Verification items for the finished model (mm, model axes). A direction names the side the tool comes from. Round coordinates to 2 decimals unless told otherwise and drop trailing zeros. Order: outer loops, then holes, each group sorted by start corner. A loop starts at its lowest first (then second) coordinate and runs counter-clockwise, first axis right, second up. Notation, with made-up numbers: M 36.25,48.25 L 66.25,48.25 A32 ccw 66.25,82.25 Z; hole C 62.25,41.25 d5. An arc over 180 degrees is marked long. Use one line per item in the form item = value. Start each with the question number.
Item 1: Tool access check on faces 1 (the flat face through (-5, -2.54, 1)), 2 (the flat face through (-22.972, -2.576, -0.787)), 3 (the flat face through (-3.175, -1, 0)). Record the directions out of +Z, -Z, +X, -X, +Y, -Y that give a thin tool (end or side, any length) a straight path to the whole face; none if there is none.
Item 2: Cross-section at A-A on z = -1.5. Enter the section's corners in (x, y) (3 decimals), then the cut area to 3 significant figures.
Item 3: Cross-section at B-B on y = -1.65. Enter the section's corners in (x, z) (1 decimal).
Item 4: Cross-section at C-C on x = -13.5. Enter the section's corners in (y, z), then the cut area to 3 significant figures.
Item 5: Cross-section at D-D on z = -24. Enter the section's corners in (x, y), then the cut area to 3 significant figures.
Item 6: Thickness scan on probe 1 along Y at (x, z) = (-6.5, 29); probe 2 along Z at (x, y) = (-2.5, -1.45) (3 decimals); probe 3 along Z at (x, y) = (-1, -2.85). Record the ranges inside material, lowest first. Write a range as [from, to].
Item 7: Go/stop test with flat-tipped pins: pin 1 Ø1.5 at (y, z) = (-2, 18) entering from -X; pin 2 Ø3 at (x, y) = (-1, -1.5) entering from -Z; pin 3 Ø1 at (x, y) = (-11, -1.5) entering from +Z. Record where each tip stops, or that it passes through.
Item 8: Release check for a two-part mould opening along Z. For faces 4 (the flat face through (-0.432, -2.576, 48.22)), 5 (the flat face through (-5, 0, 1)), 6 (the flat face through (-0.432, -2.576, -48.372)), 7 (the conical face through (19.4, -4.1, 44.8)) record: +Z half, -Z half, draft (parallel to the pull), parting line (faces both ways), or undercut.
from build123d import *

# Parameters (mm, degrees)
F0_W        = 50.8
F0_H        = 101.6
F0_R        = 1.143
F0_R_2      = 1.2394927364
F1_DEPTH    = 5.08
F2_T1_DEPTH = 127.7282991577
F2_T3_DEPTH = 76.9282991577
F3_T        = -2.54
F4_W        = 6.35
F4_H        = 19.05
F5_DEPTH    = 25.4


# Not quite as in the source:
# - a fillet or chamfer that OpenCascade refuses, or shapes differently, is made with other operations: its cross-section is extruded or revolved along the edge and cut away or added


with BuildPart() as f1:
    # F0 (on Front) → F1 (new body)
    with BuildSketch(Plane.XZ):
        with Locations((-0.076776122, -0.0760140894)):
            Rectangle(F0_W, F0_H)
        with Locations((-22.936776122, -48.2090140894)):
            Circle(F0_R, mode=Mode.SUBTRACT)
        with Locations((23.418223878, -49.0980140894)):
            Circle(F0_R, mode=Mode.SUBTRACT)
        with Locations((-23.6282116387, 48.9378400757)):
            Circle(F0_R_2, mode=Mode.SUBTRACT)
        with Locations((23.5306444928, 48.7492585503)):
            Circle(F0_R, mode=Mode.SUBTRACT)
    extrude(amount=F1_DEPTH)

    # F2: chamfer of 5.08 on 8 edges, made by hand

    # F2_s2 → F2_t1 (cut)
    with BuildSketch(Plane.XY.offset(-63.9401636683)):
        Polygon((25.323223878, -5.08), (20.243223878, 0), (25.323223878, 0), align=None)
        Polygon((-25.476776122, -5.08), (-20.396776122, 0), (-25.476776122, 0), align=None)
    extrude(amount=F2_T1_DEPTH, mode=Mode.SUBTRACT)

    # F2_s4 → F2_t3 (cut)
    with BuildSketch(Plane.YZ.offset(-38.5409257009)):
        Polygon((-5.08, 50.7239859106), (0, 45.6439859106), (0, 50.7239859106), align=None)
        Polygon((-5.08, -50.8760140894), (0, -45.7960140894), (0, -50.8760140894), align=None)
    extrude(amount=F2_T3_DEPTH, mode=Mode.SUBTRACT)

    # F2_s5 → F2_t6 (revolve, cut)
    with BuildSketch(Plane.XY.offset(48.9378400757)):
        Polygon((-22.3887189023, -5.08), (-17.3087189023, 0), (-22.3887189023, 0), align=None)
    revolve(axis=Axis((-23.6282116387, 0, 48.9378400757), (0, -1, 0)), mode=Mode.SUBTRACT)

    # F2_s7 → F2_t8 (revolve, cut)
    with BuildSketch(Plane.XY.offset(48.7492585503)):
        Polygon((24.6736444928, -5.08), (29.7536444928, 0), (24.6736444928, 0), align=None)
    revolve(axis=Axis((23.5306444928, 0, 48.7492585503), (0, -1, 0)), mode=Mode.SUBTRACT)

    # F2_s9 → F2_t10 (revolve, cut)
    with BuildSketch(Plane.XY.offset(-48.2090140894)):
        Polygon((-21.793776122, -5.08), (-16.713776122, 0), (-21.793776122, 0), align=None)
    revolve(axis=Axis((-22.936776122, 0, -48.2090140894), (0, -1, 0)), mode=Mode.SUBTRACT)

    # F2_s11 → F2_t12 (revolve, cut)
    with BuildSketch(Plane.XY.offset(-49.0980140894)):
        Polygon((24.561223878, -5.08), (29.641223878, 0), (24.561223878, 0), align=None)
    revolve(axis=Axis((23.418223878, 0, -49.0980140894), (0, -1, 0)), mode=Mode.SUBTRACT)

    # F3
    f3_openings = [f1.faces().sort_by_distance(p)[0] for p in [
        (-0.074021, -5.08, -0.083441),
    ]]
    offset(amount=F3_T, openings=f3_openings)

    # F4 (on face) → F5 (cut)
    with BuildSketch(Plane(origin=(0, 0, 0), x_dir=(-1, 0, 0), z_dir=(0, 1, 0))):
        Rectangle(F4_W, F4_H)
    extrude(amount=-F5_DEPTH, mode=Mode.SUBTRACT)


solid = f1.part
Output values:
q1.face_1 = -Y
q1.face_2 = +Z, -Z, -X, +Y
q1.face_3 = +Y, -Y
q2.outline = M -25.477,-5.08 L -21.885,-5.08 L -19.345,-2.54 L -3.175,-2.54 L -3.175,0 L -20.397,0 Z; M 3.175,-2.54 L 19.191,-2.54 L 21.731,-5.08 L 25.323,-5.08 L 20.243,0 L 3.175,0 Z
q2.area = 112 mm2
q3.outline = M -22,-43.7 A4.6 cw -18.4,-47.4 L 19.2,-47.4 A4.6 cw 21.9,-44.8 L 21.9,44.5 A4.6 cw 19.2,47.3 L -19.3,47.3 A4.7 cw -22,44.5 Z; hole M -3.2,-9.5 L 3.2,-9.5 L 3.2,9.5 L -3.2,9.5 Z
q4.outline = M -5.08,-50.88 L 0,-45.8 L 0,45.64 L -5.08,50.72 L -5.08,47.13 L -2.54,44.59 L -2.54,-44.74 L -5.08,-47.28 Z
q4.area = 257 mm2
q5.outline = M -25.48,-5.08 L -21.88,-5.08 L -19.34,-2.54 L 19.19,-2.54 L 21.73,-5.08 L 25.32,-5.08 L 20.24,0 L -20.4,0 Z
q5.area = 128 mm2
q6.probe_1 = [-2.54, 0]
q6.probe_2 = [-47.246, -9.525], [9.525, 47.094]
q6.probe_3 = [-48.65, -45.05], [44.9, 48.49]
q7.pin_1 = -23.15
q7.pin_2 = -48.8
q7.pin_3 = 47.64
q8.face_4 = +Z half
q8.face_5 = draft
q8.face_6 = -Z half
q8.face_7 = undercut
